Input: part model. Units: mm. Frame: model coordinates. Face numbers are marked on the shaded views. A direction names the side the tool comes from. Give positions to 0.01 mm unless a question says otherwise; leave off trailing zeros. Loops run counter-clockwise (first coordinate to the right, second up) from the corner with the lowest first, then second, coordinate; pieces in that order, holes last. Notation, with made-up numbers: (65, 40.5) -> (88, 40.5) arc R26 cw to (88, 74.5) -> close; hole circle Ø8 at (59, -38.5). An arc over 180 degrees is marked (long way). Use CSV: the item, a comma, the result in double quotes.
```python
from build123d import *

# Parameters (mm, degrees)
SKETCH1_W                      = 106
SKETCH1_H                      = 67.5
BOSS_EXTRUDE1_DEPTH            = 30
SKETCH2_W                      = 92.6
SKETCH2_H                      = 30
BOSS_EXTRUDE2_DEPTH            = 30
SKETCH3_W                      = 92.6
SKETCH3_H                      = 30
CUT_EXTRUDE1_DEPTH             = 30
SKETCH4_R                      = 3
CUT_EXTRUDE2_DEPTH             = 30
M3_CLEARANCE_HOLE1_D           = 3.4
M3_CLEARANCE_HOLE1_CSINK_D     = 3.45
M3_CLEARANCE_HOLE1_CSINK_ANGLE = 90
SKETCH11_R                     = 9
CUT_EXTRUDE3_DEPTH             = 2
M5_CLEARANCE_HOLE1_AT_2_COUNT  = 2
M5_CLEARANCE_HOLE1_AT_2_PITCH  = 49.748811611
M5_CLEARANCE_HOLE1_AT_3_COUNT  = 2
M5_CLEARANCE_HOLE1_AT_3_PITCH  = 46.836464196
M5_CLEARANCE_HOLE1_AT_4_COUNT  = 2
M5_CLEARANCE_HOLE1_AT_4_PITCH  = 16.77169873
M5_CLEARANCE_HOLE1_AT_5_COUNT  = 2
M5_CLEARANCE_HOLE1_AT_5_PITCH  = 16.771686167
M5_CLEARANCE_HOLE1_AT_6_COUNT  = 2
M5_CLEARANCE_HOLE1_AT_6_PITCH  = 49.748806755
M5_CLEARANCE_HOLE1_AT_7_COUNT  = 2
M5_CLEARANCE_HOLE1_AT_7_PITCH  = 49.748790588
M5_CLEARANCE_HOLE1_AT_8_COUNT  = 2
M5_CLEARANCE_HOLE1_AT_8_PITCH  = 46.836452861


with BuildPart() as part:
    # Sketch1 → Boss-Extrude1 (new body)
    with BuildSketch(Plane.XY):
        with Locations((-7.205998582, -5.840323621)):
            Rectangle(SKETCH1_W, SKETCH1_H)
    extrude(amount=BOSS_EXTRUDE1_DEPTH)

    # Sketch2 → Boss-Extrude2 (add)
    with BuildSketch(Plane.XY):
        with Locations((-13.905998582, -24.590323621)):
            Rectangle(SKETCH2_W, SKETCH2_H)
    extrude(amount=BOSS_EXTRUDE2_DEPTH)

    # Sketch3 → Cut-Extrude1 (cut)
    with BuildSketch(Plane.XY):
        with Locations((-13.905998582, -24.590323621)):
            Rectangle(SKETCH3_W, SKETCH3_H)
    extrude(amount=CUT_EXTRUDE1_DEPTH, mode=Mode.SUBTRACT)

    # Sketch4 → Cut-Extrude2 (cut)
    with BuildSketch(Plane(origin=(45.794001418, 0, 0), x_dir=(0, 0, -1), z_dir=(1, 0, 0))):
        with Locations(Location((-15, -24.590323621, 0), (0, 0, 90))):
            Circle(SKETCH4_R)
    extrude(amount=-CUT_EXTRUDE2_DEPTH, mode=Mode.SUBTRACT)

    # M3 Clearance Hole1 (through all)
    with Locations(Plane.ZY.offset(-32.394001418)):
        with Locations((7.221825407, -32.368498214), (7.221825407, -16.812149028), (22.778174593, -16.812149028), (22.778174593, -32.368498214)):
            CounterSinkHole(M3_CLEARANCE_HOLE1_D / 2, M3_CLEARANCE_HOLE1_CSINK_D / 2, counter_sink_angle=M3_CLEARANCE_HOLE1_CSINK_ANGLE)

    # Sketch11 → Cut-Extrude3 (cut)
    with BuildSketch(Plane.ZY.offset(-32.394001418)):
        with Locations((15, -24.590323621)):
            Circle(SKETCH11_R)
    extrude(amount=-CUT_EXTRUDE3_DEPTH, mode=Mode.SUBTRACT)

    # Sketch12 → M5 Clearance Hole1 (revolve, cut)
    with BuildSketch(Plane(origin=(-30.624223061, 27.909676379, 23.385849743), x_dir=(0, 0, 1), z_dir=(1, 0, 0))):
        Polygon((0, 0), (0, 67.5), (2.75, 67.5), (2.75, 0.025), (2.775, 0), align=None)
    m5_clearance_hole1 = revolve(axis=Axis((-30.624223061, 34.259676379, 23.385849743), (0, -1, 0)), mode=Mode.SUBTRACT)

    # M5 Clearance Hole1 at 2: M5 Clearance Hole1 ×2
    with Locations(*[Vector(0.9414589550934056, 0, -0.3371276254987612) * (i * M5_CLEARANCE_HOLE1_AT_2_PITCH) for i in range(1, M5_CLEARANCE_HOLE1_AT_2_COUNT)]):
        add(m5_clearance_hole1, mode=Mode.SUBTRACT)

    # M5 Clearance Hole1 at 3: M5 Clearance Hole1 ×2
    with Locations(*[(i * M5_CLEARANCE_HOLE1_AT_3_PITCH, 0, 0) for i in range(1, M5_CLEARANCE_HOLE1_AT_3_COUNT)]):
        add(m5_clearance_hole1, mode=Mode.SUBTRACT)

    # M5 Clearance Hole1 at 4: M5 Clearance Hole1 ×2
    with Locations(*[(0, 0, -i * M5_CLEARANCE_HOLE1_AT_4_PITCH) for i in range(1, M5_CLEARANCE_HOLE1_AT_4_COUNT)]):
        add(m5_clearance_hole1, mode=Mode.SUBTRACT)

    # M5 Clearance Hole1 at 5: M5 Clearance Hole1 ×2
    with Locations(*[(0, 0, -i * M5_CLEARANCE_HOLE1_AT_5_PITCH) for i in range(1, M5_CLEARANCE_HOLE1_AT_5_COUNT)]):
        add(m5_clearance_hole1, mode=Mode.SUBTRACT)

    # M5 Clearance Hole1 at 6: M5 Clearance Hole1 ×2
    with Locations(*[Vector(0.9414589495083403, 0, -0.33712764109555354) * (i * M5_CLEARANCE_HOLE1_AT_6_PITCH) for i in range(1, M5_CLEARANCE_HOLE1_AT_6_COUNT)]):
        add(m5_clearance_hole1, mode=Mode.SUBTRACT)

    # M5 Clearance Hole1 at 7: M5 Clearance Hole1 ×2
    with Locations(*[Vector(0.9414589838280241, 0, -0.3371275452547662) * (i * M5_CLEARANCE_HOLE1_AT_7_PITCH) for i in range(1, M5_CLEARANCE_HOLE1_AT_7_COUNT)]):
        add(m5_clearance_hole1, mode=Mode.SUBTRACT)

    # M5 Clearance Hole1 at 8: M5 Clearance Hole1 ×2
    with Locations(*[(i * M5_CLEARANCE_HOLE1_AT_8_PITCH, 0, 0) for i in range(1, M5_CLEARANCE_HOLE1_AT_8_COUNT)]):
        add(m5_clearance_hole1, mode=Mode.SUBTRACT)


solid = part.part
```
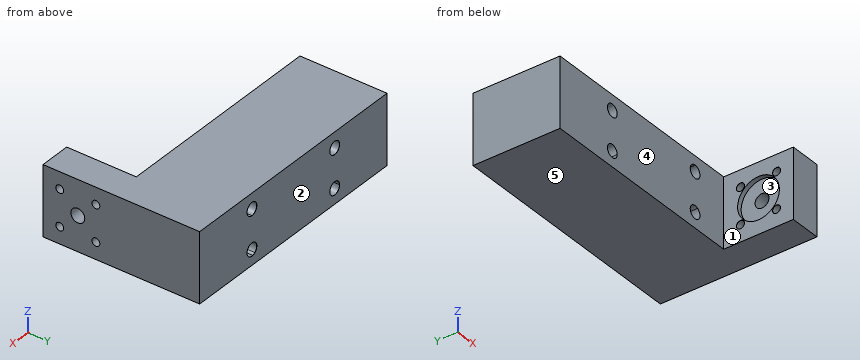
1) Section query D-D (x = 37.5). Return loops of the section in (y, z).
From the geometry:
outline,"(-39.59, 0) -> (27.91, 0) -> (27.91, 30) -> (-39.59, 30) -> close; hole circle Ø3.4 at (-32.37, 7.22); hole circle Ø3.4 at (-32.37, 22.78); hole circle Ø6 at (-24.59, 15); hole circle Ø3.4 at (-16.81, 7.22); hole circle Ø3.4 at (-16.81, 22.78)"
2) Mould query, pull axis Z, two halves, no side actions, for the marked faces 3, 4 and 5. Classes: pulls with the +Z half, pulls with the -Z half, needs draft (parallel to the pull), parting line crosses it, or undercut.
From the geometry:
face 3,"undercut"
face 4,"needs draft"
face 5,"pulls with the -Z half"
3) Reachability of the marked faces 1 and 2 from +Z, -Z, +X, -X, +Y, -Y: full face, straight path, thin tool, end or side. Return the list, or none.
From the geometry:
face 1,"+Z, -Z, -X, -Y"
face 2,"+Z, -Z, +X, -X, +Y"
4) Ray query, line 1 (X direction, y = 5, z = 6.25); line 2 (Z direction, x = -29, y = -7.5); line 3 (Y direction, x = 33.1, z = 15). Return the intervals inside material, ascending.
From the geometry:
line 1,"x = -60.21 to -33.35, -27.9 to 13.49, 18.94 to 45.79"
line 2,"z = 0 to 4.4, 8.83 to 21.17, 25.6 to 30"
line 3,"y = -39.59 to -33.59, -15.59 to 27.91"
5) Section query B-B (y = 3). Return loops of the section in (x, z), then the cut area to 3 significant figures.
From the geometry:
outline,"(-60.21, 0) -> (45.79, 0) -> (45.79, 30) -> (-60.21, 30) -> close; hole (-33.37, 6.61) arc R2.75 ccw to (-27.87, 6.61) arc R2.75 ccw to start; hole circle Ø5.5 at (-30.62, 23.39); hole (14.55, 4.42) arc R2.75 ccw to (15.73, 3.91) arc R2.75 ccw to (17.63, 8.97) arc R2.75 ccw to start; hole (16.21, 20.64) arc R2.75 ccw to (16.21, 26.14) arc R2.75 ccw to start"
area,"3,080 mm^2"
6) Section query A-A (z = 15). Return loops of the section in (x, y).
From the geometry:
outline,"(-60.21, -9.59) -> (32.39, -9.59) -> (32.39, -15.59) -> (34.39, -15.59) -> (34.39, -21.59) -> (45.79, -21.59) -> (45.79, 27.91) -> (-60.21, 27.91) -> close; (32.39, -39.59) -> (45.79, -39.59) -> (45.79, -27.59) -> (34.39, -27.59) -> (34.39, -33.59) -> (32.39, -33.59) -> close"
7) Section query C-C (y = -23). Return loops of the section in (x, z), then the cut area to 3 significant figures.
From the geometry:
outline,"(32.39, 0) -> (45.79, 0) -> (45.79, 12.46) -> (34.39, 12.46) -> (34.39, 6.14) -> (32.39, 6.14) -> close; (32.39, 23.86) -> (34.39, 23.86) -> (34.39, 17.54) -> (45.79, 17.54) -> (45.79, 30) -> (32.39, 30) -> close"
area,"309 mm^2"
8) Contact query for flat-ended pins moving along their axis: pin 1 (3 mm diameter, centred on y = -32.37, z = 7.22, fed in from -X); pin 2 (4 mm diameter, centred on y = -32.37, z = 22.78, fed in from -X); pin 3 (9 mm diameter, centred on x = 5.5, z = 16, fed in from -Y). Output: stop coordinate, or through.
From the geometry:
pin 1,"passes through"
pin 2,"stops at x = 32.39"
pin 3,"stops at y = -9.59"
